from build123d import *

# Parameters (mm, degrees)
SKETCH1_W           = 15
SKETCH1_H           = 45
BOSS_EXTRUDE1_DEPTH = 2.2
SKETCH1_3_W         = 20
SKETCH1_3_H         = 50
SKETCH1_3_W_2       = 15
SKETCH1_3_H_2       = 45
BOSS_EXTRUDE2_DEPTH = 2.5
SKETCH1_4_W         = 20
SKETCH1_4_H         = 50
SKETCH1_4_R         = 4.1
BOSS_EXTRUDE3_DEPTH = 2.5
FILLET1_R           = 2
SKETCH1_5_R         = 3.15
BOSS_EXTRUDE4_DEPTH = 2.5
FILLET2_R           = 10
SKETCH2_R           = 3.15
CUT_EXTRUDE1_DEPTH  = 4
SKETCH3_OUTSIDE_W   = 50.164
SKETCH3_OUTSIDE_H   = 169.464
CUT_EXTRUDE2_DEPTH  = 115.845504919


with BuildPart() as part:
    # Sketch1 → Boss-Extrude1 (new body)
    with BuildSketch(Plane(origin=(0, 0, 0), x_dir=(1, 0, 0), z_dir=(0, 1, 0))):
        Rectangle(SKETCH1_W, SKETCH1_H)
        with BuildLine():
            ThreePointArc((-3.894544437, -4.023993492), (-5.599998379, 0.004260474), (-3.88841703, 4.029914763))
            Line((-3.88841703, 4.029914763), (-3.88841703, 8.505312122))
            ThreePointArc((-3.88841703, 8.505312122), (-3.870707724, 8.925763598), (-3.817705253, 9.343236712))
            Line((-3.817705253, 9.343236712), (-2.664584371, 16.126741161))
            ThreePointArc((-2.664584371, 16.126741161), (-2.610617779, 16.555799687), (-2.593926654, 16.987916591))
            ThreePointArc((-2.593926654, 16.987916591), (0, 19.6), (2.606045235, 17.000007028))
            ThreePointArc((2.606045235, 17.000007028), (2.623754541, 16.579555552), (2.676757012, 16.162082438))
            Line((2.676757012, 16.162082438), (3.829877895, 9.378577989))
            ThreePointArc((3.829877895, 9.378577989), (3.882880366, 8.961104875), (3.900589672, 8.540653399))
            Line((3.900589672, 8.540653399), (3.900589672, 4.018133922))
            ThreePointArc((3.900589672, 4.018133922), (5.157678846, 2.181364004), (5.6, 0))
            ThreePointArc((5.6, 0), (5.156037667, -2.185240393), (3.894544437, -4.023993492))
            Line((3.894544437, -4.023993492), (3.894544437, -8.540646372))
            ThreePointArc((3.894544437, -8.540646372), (3.876835131, -8.961097847), (3.82383266, -9.378570962))
            Line((3.82383266, -9.378570962), (2.670711777, -16.16207541))
            ThreePointArc((2.670711777, -16.16207541), (2.617709306, -16.579548524), (2.6, -17))
            ThreePointArc((2.6, -17), (0, -19.6), (-2.6, -17))
            ThreePointArc((-2.6, -17), (-2.617709306, -16.579548524), (-2.670711777, -16.16207541))
            Line((-2.670711777, -16.16207541), (-3.82383266, -9.378570962))
            ThreePointArc((-3.82383266, -9.378570962), (-3.876835131, -8.961097847), (-3.894544437, -8.540646372))
            Line((-3.894544437, -8.540646372), (-3.894544437, -4.023993492))
        make_face(mode=Mode.SUBTRACT)
    extrude(amount=-BOSS_EXTRUDE1_DEPTH)

    # Sketch1<3> → Boss-Extrude2 (add)
    # profile 1 of 2: a face of its own
    with BuildSketch(Plane(origin=(0, 0, 0), x_dir=(1, 0, 0), z_dir=(0, 1, 0))):
        Rectangle(SKETCH1_3_W, SKETCH1_3_H)
        Rectangle(SKETCH1_3_W_2, SKETCH1_3_H_2, mode=Mode.SUBTRACT)
    # profile 2 of 2: a face of its own
    with BuildSketch(Plane(origin=(0, 0, 0), x_dir=(1, 0, 0), z_dir=(0, 1, 0))):
        Rectangle(SKETCH1_3_W_2, SKETCH1_3_H_2)
        with BuildLine():
            ThreePointArc((-3.894544437, -4.023993492), (-5.599998379, 0.004260474), (-3.88841703, 4.029914763))
            Line((-3.88841703, 4.029914763), (-3.88841703, 8.505312122))
            ThreePointArc((-3.88841703, 8.505312122), (-3.870707724, 8.925763598), (-3.817705253, 9.343236712))
            Line((-3.817705253, 9.343236712), (-2.664584371, 16.126741161))
            ThreePointArc((-2.664584371, 16.126741161), (-2.610617779, 16.555799687), (-2.593926654, 16.987916591))
            ThreePointArc((-2.593926654, 16.987916591), (0, 19.6), (2.606045235, 17.000007028))
            ThreePointArc((2.606045235, 17.000007028), (2.623754541, 16.579555552), (2.676757012, 16.162082438))
            Line((2.676757012, 16.162082438), (3.829877895, 9.378577989))
            ThreePointArc((3.829877895, 9.378577989), (3.882880366, 8.961104875), (3.900589672, 8.540653399))
            Line((3.900589672, 8.540653399), (3.900589672, 4.018133922))
            ThreePointArc((3.900589672, 4.018133922), (5.157678846, 2.181364004), (5.6, 0))
            ThreePointArc((5.6, 0), (5.156037667, -2.185240393), (3.894544437, -4.023993492))
            Line((3.894544437, -4.023993492), (3.894544437, -8.540646372))
            ThreePointArc((3.894544437, -8.540646372), (3.876835131, -8.961097847), (3.82383266, -9.378570962))
            Line((3.82383266, -9.378570962), (2.670711777, -16.16207541))
            ThreePointArc((2.670711777, -16.16207541), (2.617709306, -16.579548524), (2.6, -17))
            ThreePointArc((2.6, -17), (0, -19.6), (-2.6, -17))
            ThreePointArc((-2.6, -17), (-2.617709306, -16.579548524), (-2.670711777, -16.16207541))
            Line((-2.670711777, -16.16207541), (-3.82383266, -9.378570962))
            ThreePointArc((-3.82383266, -9.378570962), (-3.876835131, -8.961097847), (-3.894544437, -8.540646372))
            Line((-3.894544437, -8.540646372), (-3.894544437, -4.023993492))
        make_face(mode=Mode.SUBTRACT)
    extrude(amount=-BOSS_EXTRUDE2_DEPTH)

    # Sketch1<4> → Boss-Extrude3 (add)
    with BuildSketch(Plane(origin=(0, 0, 0), x_dir=(1, 0, 0), z_dir=(0, 1, 0))):
        Rectangle(SKETCH1_4_W, SKETCH1_4_H)
        with Locations(Location((0, 0, 0), (0, 0, 270))):
            Circle(SKETCH1_4_R, mode=Mode.SUBTRACT)
    extrude(amount=BOSS_EXTRUDE3_DEPTH)

    # Fillet1
    fillet1_edges = [part.edges().sort_by_distance(p)[0] for p in [
        (-3.88841703, -1.25, -4.029914763),
        (-3.894544437, -1.25, 4.023993492),
        (3.894544437, -1.25, 4.023993492),
        (3.900589672, -1.25, -4.018133922),
    ]]
    fillet(fillet1_edges, radius=FILLET1_R)

    # Sketch1<5> → Boss-Extrude4 (add, symmetric)
    with BuildSketch(Plane(origin=(0, 0, 0), x_dir=(1, 0, 0), z_dir=(0, 1, 0))):
        with BuildLine():
            ThreePointArc((-10, 104.3), (0, 114.3), (10, 104.3))
            Line((10, 104.3), (10, 25))
            Line((10, 25), (-10, 25))
            Line((-10, 25), (-10, 104.3))
        make_face()
        with Locations(Location((0, 104.3, 0), (0, 0, 270))):
            Circle(SKETCH1_5_R, mode=Mode.SUBTRACT)
    extrude(amount=BOSS_EXTRUDE4_DEPTH, both=True)

    # Fillet2
    fillet2_edges = [part.edges().sort_by_distance(p)[0] for p in [
        (10, 0, 25),
        (-10, 0, 25),
    ]]
    fillet(fillet2_edges, radius=FILLET2_R - 0.0001)  # a hair under: the kernel refuses the full size

    # Sketch2 → Cut-Extrude1 (cut)
    # profile 1 of 8: a face of its own
    with BuildSketch(Plane.XZ.offset(2.5)):
        with Locations(Location((0, -104.3, 0), (0, 0, 90))):
            Circle(SKETCH2_R)
    # profile 2 of 8: a face of its own
    with BuildSketch(Plane.XZ.offset(2.5)):
        Polygon((5.973502692, -72.744870683), (-2.986751346, -67.571665602), (-2.986751346, -77.918075763), align=None)
        Polygon((5.773502692, -72.744870683), (-2.886751346, -67.744870683), (-2.886751346, -77.744870683), align=None, mode=Mode.SUBTRACT)
    # profile 3 of 8: a face of its own
    with BuildSketch(Plane.XZ.offset(2.5)):
        Polygon((5.973502692, -56.744870683), (-2.986751346, -51.571665602), (-2.986751346, -61.918075763), align=None)
        Polygon((5.773502692, -56.744870683), (-2.886751346, -51.744870683), (-2.886751346, -61.744870683), align=None, mode=Mode.SUBTRACT)
    # profile 4 of 8: a face of its own
    with BuildSketch(Plane.XZ.offset(2.5)):
        Polygon((5.973502692, -40.744870683), (-2.986751346, -35.571665602), (-2.986751346, -45.918075763), align=None)
        Polygon((5.773502692, -40.744870683), (-2.886751346, -35.744870683), (-2.886751346, -45.744870683), align=None, mode=Mode.SUBTRACT)
    # profile 5 of 8: a face of its own
    with BuildSketch(Plane.XZ.offset(2.5)):
        Polygon((5.973502692, -24.744870683), (-2.986751346, -19.571665602), (-2.986751346, -29.918075763), align=None)
        Polygon((5.773502692, -24.744870683), (-2.886751346, -19.744870683), (-2.886751346, -29.744870683), align=None, mode=Mode.SUBTRACT)
    # profile 6 of 8: a face of its own
    with BuildSketch(Plane.XZ.offset(2.5)):
        Polygon((-3.086751346, -64.744870683), (5.873502692, -59.571665602), (5.873502692, -69.918075763), align=None)
        Polygon((5.773502692, -69.744870683), (-2.886751346, -64.744870683), (5.773502692, -59.744870683), align=None, mode=Mode.SUBTRACT)
    # profile 7 of 8: a face of its own
    with BuildSketch(Plane.XZ.offset(2.5)):
        Polygon((-3.086751346, -48.744870683), (5.873502692, -43.571665602), (5.873502692, -53.918075763), align=None)
        Polygon((5.773502692, -53.744870683), (-2.886751346, -48.744870683), (5.773502692, -43.744870683), align=None, mode=Mode.SUBTRACT)
    # profile 8 of 8: a face of its own
    with BuildSketch(Plane.XZ.offset(2.5)):
        Polygon((-3.086751346, -32.744870683), (5.873502692, -27.571665602), (5.873502692, -37.918075763), align=None)
        Polygon((5.773502692, -37.744870683), (-2.886751346, -32.744870683), (5.773502692, -27.744870683), align=None, mode=Mode.SUBTRACT)
    extrude(amount=-CUT_EXTRUDE1_DEPTH, mode=Mode.SUBTRACT)

    # Sketch3 outside → Cut-Extrude2 (cut, through all)
    with BuildSketch(Plane.XZ.offset(2.5)):
        with Locations((0, -44.65)):
            Rectangle(SKETCH3_OUTSIDE_W, SKETCH3_OUTSIDE_H)
        with BuildLine():
            Line((10, -50.039570793), (10, 15))
            ThreePointArc((10, 15), (7.071067812, 22.071067812), (0, 25))
            ThreePointArc((0, 25), (-7.071067812, 22.071067812), (-10, 15))
            Line((-10, 15), (-10, -52.98511299))
            add(Edge.make_bspline(
                [(-10, -52.98511299), (-9.762519387, -55.301766927), (-9.181616668, -60.883726896), (-8.247873188, -69.548054482), (-7.214243072, -78.778305336), (-6.212768932, -87.409094774), (-5.257188729, -95.387335619), (-4.359016041, -102.663786405), (-3.588431315, -108.744280233), (-3.115741639, -112.393973299), (-2.923840172, -113.863009916)],
                knots=[0.870609711, 0.870609711, 0.870609711, 0.870609711, 0.882031045, 0.898133678, 0.913348978, 0.927582736, 0.940746445, 0.952757055, 0.963540146, 0.970806103, 0.970806103, 0.970806103, 0.970806103], degree=3))
            ThreePointArc((-2.923840172, -113.863009916), (-0.162206263, -114.29868437), (2.612106393, -113.952818251))
            add(Edge.make_bspline(
                [(2.612106393, -113.952818251), (2.807985487, -112.453854191), (3.284635603, -108.774231255), (4.059016041, -102.663786405), (4.957188729, -95.387335619), (5.912768932, -87.409094774), (6.914243072, -78.778305336), (7.947873188, -69.548054482), (8.987364419, -59.902479724), (9.66619931, -53.338446984), (10, -50.039570793)],
                knots=[0.029045831, 0.029045831, 0.029045831, 0.029045831, 0.036459854, 0.047242945, 0.059253555, 0.072417264, 0.086651022, 0.101866322, 0.117968955, 0.134230571, 0.134230571, 0.134230571, 0.134230571], degree=3))
        make_face(mode=Mode.SUBTRACT)
    extrude(amount=-CUT_EXTRUDE2_DEPTH, mode=Mode.SUBTRACT)


solid = part.part
Build history of the part. All positions in model axes, mm. A direction names the side the tool comes from. Coordinates: 2 decimals unless noted, no trailing zeros. Write each loop counter-clockwise with the first axis right and the second up, starting at its lowest first coordinate (ties: lowest second). Pieces come first, ordered by that corner, then holes. Notation, with made-up numbers: (-17, 38.25) -> (34, 38.25) arc R20 ccw to (34, 62.25) -> close; hole circle Ø6 at (89.25, -38). An arc over 180 degrees is marked (long way). Use CSV: the item, a comma, the result in double quotes. Start each with the question number.
Q1. Cut at B-B, the plane y = -1.2. State how many separate pieces and enclosed holes the cut face has, then the cut area to 3 significant figures.
Q2. Cut at A-A, the plane z = -6. List the corners of the cut face in (x, y).
Q3. Flat gauge pins, fed straight in: pin 1 Ø1.2 at (y, z) = (-0.5, -65.5) entering from -X; pin 2 Ø3 at (y, z) = (0, -83.5) entering from -X; pin 3 Ø1.5 at (x, y) = (-1, -1.5) entering from -Z. Where does each tip first touch, or does it go through?
Q4. 3-axis set-ups, long thin cutter, end or side, ignore diameter. For faces 1 (the flat face through (-3.24, -1.23, 12.82)), 2 (the flat face through (2, -2.5, -33)): which of +Z, -Z, +X, -X, +Y, -Y reach the whole face in a straight line?
Q5. Drill centre lines: probe 1 along X at (y, z) = (1.55, -0.5); probe 2 along X at (y, z) = (-1.5, -78.5); probe 3 along X at (y, z) = (-0.7, -1.5). Where is each one in solid material? Low to high.
Q6. Pull direction Z, two halves, no side cores. Call faces 3 (the cylindrical face through (-0.2, 0, -114.3)), 4 (the flat face through (3.255, -1.232, 12.723)), 5 (the flat face through (0, -2.5, -46)): released by +Z, released by -Z, zero draft, split by the parting line, or undercut.
Checked values:
1,separate pieces,"8"
1,enclosed holes,"9"
1,area,"1,970 mm²"
2,outline,"(-10, -2.5) -> (-3.89, -2.5) -> (-3.89, 0) -> (3.9, 0) -> (3.9, -2.5) -> (10, -2.5) -> (10, 2.5) -> (-10, 2.5) -> close"
3,pin 1,"stops at x = -8.75"
3,pin 2,"stops at x = -6.84"
3,pin 3,"stops at z = -114.3"
4,face 1,"-Y"
4,face 2,"+Z, -Z, +X, -X, -Y"
5,probe 1,"x = -10 to -4.07, 4.07 to 10"
5,probe 2,"x = -7.24 to 6.94"
5,probe 3,"x = -10 to -5.4, 5.4 to 10"
6,face 3,"released by -Z"
6,face 4,"undercut"
6,face 5,"zero draft"
